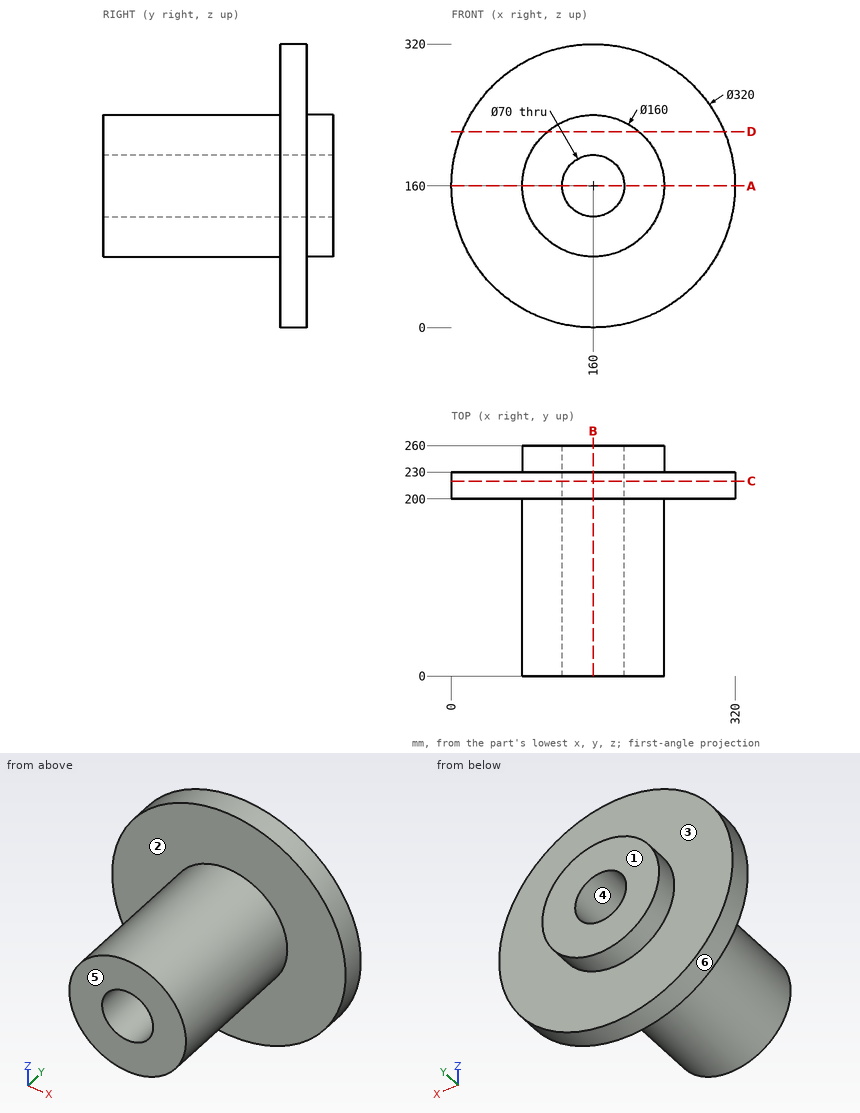
Geometry check sheet. Reference: drawing and pictorial views, mm from the part's lowest x, y, z. A direction names the side the tool comes from. Round coordinates to 2 decimals unless told otherwise and drop trailing zeros. Loops run counter-clockwise (first coordinate to the right, second up) from the corner with the lowest first, then second, coordinate; pieces in that order, holes last. Notation, with made-up numbers: (88, -38.5) -> (147, -38.5) arc R20 cw to (147, -18.5) -> close; hole circle Ø3 at (19.25, 80). An arc over 180 degrees is marked (long way). Answer as a JSON object with one key per item and string values. Group by question number.
Item 1: Depth check by flat-ended pin: pin 1 Ø8 at (y, z) = (160, 203.5) entering from +X; pin 2 Ø1.5 at (x, y) = (117.5, 208.5) entering from -Z; pin 3 Ø2 at (y, z) = (207.5, 129) entering from -X. Enter the tip coordinate at first touch or a pass-through.
Item 2: Thickness scan on line 1 along X through (y, z) = (199, 160); line 2 along Y through (x, z) = (82.5, 34.5); line 3 along Z through (x, y) = (184, 134.5). Record the ranges inside material, lowest first.
Item 3: Release check for a two-part mould opening along X. For the marked faces 4, 5 and 6 record: pulls with the +X half, pulls with the -X half, needs draft (parallel to the pull), parting line crosses it, or undercut.
Item 4: Set-up check for the marked faces 1, 2 and 3: record each of +Z, -Z, +X, -X, +Y, -Y from which the full face is reachable in a straight line by a thin tool's end or side.
Item 5: Cross-section at A-A, the plane z = 160. Record the cut outline in (x, y).
Item 6: Cross-section at D-D, the plane z = 221. Record the cut outline in (x, y), plus the area to 3 significant figures.
Item 7: Cross-section at C-C, the plane y = 220. Record the cut outline in (x, z).
Item 8: Cross-section at B-B, the plane x = 160. Record the cut outline in (y, z), plus the area to 3 significant figures.
Determined:
{
 "1": {"pin 1": "stops at x = 229.57", "pin 2": "stops at z = 5.54", "pin 3": "stops at x = 2.84"},
 "2": {"line 1": "x = 80 to 125, 195 to 240", "line 2": "y = 200 to 230", "line 3": "z = 83.68 to 134.52, 185.48 to 236.32"},
 "3": {"face 4": "undercut", "face 5": "needs draft", "face 6": "parting line crosses it"},
 "4": {"face 1": "+Z, -Z, +X, -X, +Y", "face 2": "-Y", "face 3": "+Y"},
 "5": {"outline": "(0, 200) -> (80, 200) -> (80, 0) -> (125, 0) -> (125, 260) -> (80, 260) -> (80, 230) -> (0, 230) -> close; (195, 0) -> (240, 0) -> (240, 200) -> (320, 200) -> (320, 230) -> (240, 230) -> (240, 260) -> (195, 260) -> close"},
 "6": {"outline": "(12.08, 200) -> (108.24, 200) -> (108.24, 0) -> (211.76, 0) -> (211.76, 200) -> (307.92, 200) -> (307.92, 230) -> (211.76, 230) -> (211.76, 260) -> (108.24, 260) -> (108.24, 230) -> (12.08, 230) -> close", "area": "32,700 mm²"},
 "7": {"outline": "circle Ø320 at (160, 160); hole circle Ø70 at (160, 160)"},
 "8": {"outline": "(0, 80) -> (200, 80) -> (200, 0) -> (230, 0) -> (230, 80) -> (260, 80) -> (260, 125) -> (0, 125) -> close; (0, 195) -> (260, 195) -> (260, 240) -> (230, 240) -> (230, 320) -> (200, 320) -> (200, 240) -> (0, 240) -> close", "area": "28,200 mm²"}
}
